Check sheet for the modelled part. Datum: model origin and axes. Units: mm. A direction names the side the tool comes from. Round coordinates to 2 decimals unless told otherwise and drop trailing zeros. Write each loop counter-clockwise with the first axis right and the second up, starting at its lowest first coordinate (ties: lowest second). Pieces come first, ordered by that corner, then holes.
Solid Edge part; units mm, degrees
sketch "Sketch1" plane through (0, 0, 0) normal (1, 0, 0) x (0, 1, 0)
  circle A0 centre (0, 0) radius 8.5
  circle A1 centre (10, 6) radius 2
  circle A2 centre (-10, -10) radius 2
  line L0 (40, 15) -> (40, 12.2)
  line L1 (40, 12.2) -> (43, 12.2)
  line L2 (43, 12.2) -> (43, -7.8)
  line L3 (43, -7.8) -> (40, -7.8)
  line L4 (40, -7.8) -> (40, -15)
  line L5 (40, -15) -> (-40, -15)
  line L6 (-40, -15) -> (-40, -7.8)
  line L7 (-40, -7.8) -> (-43, -7.8)
  line L8 (-43, -7.8) -> (-43, 12.2)
  line L9 (-43, 12.2) -> (-40, 12.2)
  line L10 (-40, 12.2) -> (-40, 15)
  line L11 (-40, 15) -> (40, 15)
  dimension "D1" = 40
  dimension "D2" = 40
  dimension "D3" = 43
  dimension "D4" = 40
extrude "Protrusion1" add sketch "Sketch1" against normal blind 3
properties material "Acier"
1. Release check for a two-part mould opening along Y. For faces 6 (the flat face through (-1, -40, -11)), 7 (the cylindrical face through (-1.479, 4.57, 7.167)), 8 (the flat face through (-3, -10, 0)) record: released by +Y, released by -Y, zero draft, split by the parting line, or undercut.
2. Sectioned sample at A-A, the plane z = -10. Enter the section's corners in (x, y).
3. Set-up check for faces 1 (the flat face through (-1, 40, 14)), 2 (the flat face through (-1, 42, -7.8)), 3 (the flat face through (-1, -41, -7.8)), 4 (the flat face through (-1, -40, 14)), 5 (the flat face through (-1, -43, 2)): record each of +Z, -Z, +X, -X, +Y, -Y from which the full face is reachable in a straight line by a thin tool's end or side.
4. Scan lines: line 1 along Y through (x, z) = (-2.7, 5.5); line 2 along Y through (x, z) = (-1.8, 0.25); line 3 along Z through (x, y) = (-1.95, 10). Record each from-to range of solid material in increasing order.
5. Go/stop test with flat-tipped pins: pin 1 (0.8 mm diameter, centred on x = -1, z = 13.5, fed in from +Y); pin 2 (1.5 mm diameter, centred on x = -1.5, z = -12.5, fed in from -Y); pin 3 (3.5 mm diameter, centred on y = -10, z = -10, fed in from +X). Record where each tip stops, or that it passes through.
6. Sectioned sample at B-B, the plane y = -10. Enter the section's corners in (x, z), plus the area to 3 significant figures.
7. Sectioned sample at D-D, the plane z = 6. Enter the section's corners in (x, y).
8. Sectioned sample at C-C, the plane x = -2. Enter the section's corners in (y, z).
Computed values:
1. face 6: released by -Y
1. face 7: undercut
1. face 8: zero draft
2. outline: (-3, -40) - (0, -40) - (0, -12) - (-3, -12) - close; (-3, -8) - (0, -8) - (0, 40) - (-3, 40) - close
3. face 1: +Z, +X, -X, +Y
3. face 2: -Z, +X, -X, +Y
3. face 3: -Z, +X, -X, -Y
3. face 4: +Z, +X, -X, -Y
3. face 5: +Z, -Z, +X, -X, -Y
4. line 1: y = -43 to -6.48, 6.48 to 8.06, 11.94 to 43
4. line 2: y = -43 to -8.5, 8.5 to 43
4. line 3: z = -15 to 4, 8 to 15
5. pin 1: stops at y = 40
5. pin 2: stops at y = -40
5. pin 3: passes through
6. outline: (-3, -15) - (0, -15) - (0, -12) - (-3, -12) - close; (-3, -8) - (0, -8) - (0, 15) - (-3, 15) - close
6. area: 78.0 mm2
7. outline: (-3, -43) - (0, -43) - (0, -6.02) - (-3, -6.02) - close; (-3, 6.02) - (0, 6.02) - (0, 8) - (-3, 8) - close; (-3, 12) - (0, 12) - (0, 43) - (-3, 43) - close
8. outline: (-43, -7.8) - (-40, -7.8) - (-40, -15) - (40, -15) - (40, -7.8) - (43, -7.8) - (43, 12.2) - (40, 12.2) - (40, 15) - (-40, 15) - (-40, 12.2) - (-43, 12.2) - close; hole circle Ø4 at (-10, -10); hole circle Ø17 at (0, 0); hole circle Ø4 at (10, 6)
